Check sheet for the modelled part. Datum: model origin and axes. Units: mm. Face numbers are marked on the shaded views. A direction names the side the tool comes from. Give positions to 0.01 mm unless a question says otherwise; leave off trailing zeros. Order: outer loops, then holes, each group sorted by start corner. A loop starts at its lowest first (then second) coordinate and runs counter-clockwise, first axis right, second up.
Item 1: Release check for a two-part mould opening along X. For the marked faces 1 and 2 record: released by +X, released by -X, zero draft, split by the parting line, or undercut.
Item 2: Material ranges on line 1 along Y through (x, z) = (10, 1.7); line 2 along X through (y, z) = (-0.5, 1.25); line 3 along X through (y, z) = (2, 2.25), recorded low to high.
Item 3: Sectioned sample at C-C on y = 0. Count the separate pieces of the cut face and the enclosed holes in it, and give its area (3 significant figures).
Item 4: Gauge pin test, flat ends, axial feed: P1, Ø0.5, axis at x = 2.5, z = 1.5, coming from the +Y side; P2, Ø4, axis at x = 10, y = 0, coming from the +Z side; P3, Ø0.9, axis at x = 6.5, z = 2, coming from the -Y side. Record the tip position at first contact, or that the pin passes through.
Item 5: Sectioned sample at A-A on x = -1.5. Record the boundary of the cut face in (y, z).
Item 6: Sectioned sample at D-D on z = 6.25. Record the boundary of the cut face in (x, y).
Item 7: Sectioned sample at B-B on x = 10. Record the boundary of the cut face in (y, z).
Item 8: Access from +Z, -Z, +X, -X, +Y, -Y to the whole of each face (thin tool, end or side, straight path). Record for the marked faces 3 and 4.
from build123d import *

# Parameters (mm, degrees)
SKETCH_W        = 30
SKETCH_H        = 15
PAD_DEPTH       = 1
SKETCH001_W     = 27.8
SKETCH001_H     = 12.8
SKETCH001_W_2   = 25.8
SKETCH001_H_2   = 10.8
PAD001_DEPTH    = 1.8
SKETCH002_W     = 8
SKETCH002_H     = 1.1
PAD002_DEPTH    = 6
SKETCH003_W     = 5.2
SKETCH003_H     = 1
POCKET_DEPTH    = 28.901
SKETCH004_R     = 2.6
SKETCH004_R_2   = 1.6
PAD003_DEPTH    = 2.4
SKETCH005_W     = 10
SKETCH005_H     = 6
POCKET001_DEPTH = 5
CHAMFER_SIZE    = 0.5
CHAMFER001_SIZE = 0.5
CHAMFER002_SIZE = 0.5


with BuildPart() as part:
    # Sketch → Pad (new body)
    with BuildSketch(Plane.XY):
        Rectangle(SKETCH_W, SKETCH_H)
    extrude(amount=PAD_DEPTH)

    # Sketch001 → Pad001 (new body)
    with BuildSketch(Plane.XY.offset(1)):
        Rectangle(SKETCH001_W, SKETCH001_H)
        Rectangle(SKETCH001_W_2, SKETCH001_H_2, mode=Mode.SUBTRACT)
    extrude(amount=PAD001_DEPTH)

    # Sketch002 → Pad002 (new body)
    with BuildSketch(Plane.XY.offset(1)):
        with Locations((0, -6.95)):
            Rectangle(SKETCH002_W, SKETCH002_H)
    extrude(amount=PAD002_DEPTH)

    # Sketch003 → Pocket (cut, through all)
    with BuildSketch(Plane(origin=(-13.9, 0, 0), x_dir=(0, -1, 0), z_dir=(-1, 0, 0))):
        with Locations((0, 1.5)):
            Rectangle(SKETCH003_W, SKETCH003_H)
    extrude(amount=-POCKET_DEPTH, mode=Mode.SUBTRACT)

    # Sketch004 → Pad003 (new body)
    with BuildSketch(Plane.XY.offset(1)):
        with Locations((-10, 0)):
            Circle(SKETCH004_R)
        with Locations((-10, 0)):
            Circle(SKETCH004_R_2, mode=Mode.SUBTRACT)
        with Locations((10, 0)):
            Circle(SKETCH004_R)
        with Locations((10, 0)):
            Circle(SKETCH004_R_2, mode=Mode.SUBTRACT)
    extrude(amount=PAD003_DEPTH)

    # Sketch005 → Pocket001 (cut)
    with BuildSketch(Plane(origin=(0, 0, 0), x_dir=(1, 0, 0), z_dir=(0, 0, -1))):
        with Locations((0, -2)):
            Rectangle(SKETCH005_W, SKETCH005_H)
    extrude(amount=-POCKET001_DEPTH, mode=Mode.SUBTRACT)

    # Chamfer
    chamfer_edges = [part.edges().sort_by_distance(p)[0] for p in [
        (-11.6, 0, 3.4),
        (8.4, 0, 3.4),
    ]]
    chamfer(chamfer_edges, length=CHAMFER_SIZE)

    # Chamfer001
    chamfer001_edges = [part.edges().sort_by_distance(p)[0] for p in [
        (-13.9, 6.4, 1.9),
        (-13.9, 0, 2.8),
        (-13.9, -6.4, 1.9),
        (13.9, 6.4, 1.9),
        (13.9, 0, 2.8),
        (13.9, -6.4, 1.9),
    ]]
    chamfer(chamfer001_edges, length=CHAMFER001_SIZE)

    # Chamfer002
    chamfer002_edges = [part.edges().sort_by_distance(p)[0] for p in [
        (-5, 2, 0),
        (0, 5, 0),
        (5, 2, 0),
        (0, -1, 0),
    ]]
    chamfer(chamfer002_edges, length=CHAMFER002_SIZE)


solid = part.part
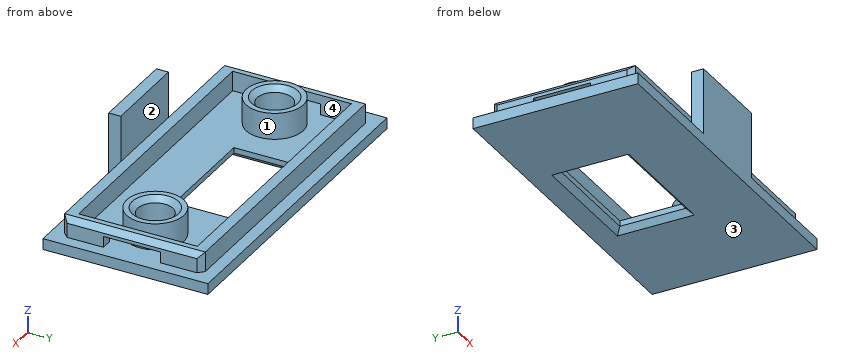
Report:
1. face 1: undercut
1. face 2: zero draft
2. line 1: y = -6.4 to -5.4, -2.6 to -1.6, 1.6 to 2.6, 5.4 to 6.4
2. line 2: x = -12.55 to -11.52, -8.48 to -7.45, 7.45 to 8.48, 11.52 to 12.55
2. line 3: x = -13.9 to -12.9, -11.66 to -8.34, 8.34 to 11.66, 12.9 to 13.9
3. separate pieces: 4
3. enclosed holes: 0
3. area: 30.2 mm2
4. P1: stops at y = 6.4
4. P2: stops at z = 3.3
4. P3: stops at y = -6.4
5. outline: (-7.5, 0) - (-1.5, 0) - (-1, 0.5) - (-1, 1) - (-5.4, 1) - (-5.4, 2.8) - (-6.4, 2.8) - (-6.4, 7) - (-7.5, 7) - close; (5, 0.5) - (5.5, 0) - (7.5, 0) - (7.5, 1) - (6.4, 1) - (6.4, 2.8) - (5.4, 2.8) - (5.4, 1) - (5, 1) - close
6. outline: (-4, -7.5) - (4, -7.5) - (4, -6.4) - (-4, -6.4) - close
7. outline: (-7.5, 0) - (7.5, 0) - (7.5, 1) - (6.4, 1) - (6.4, 2.8) - (5.4, 2.8) - (5.4, 1) - (2.6, 1) - (2.6, 3.4) - (2.1, 3.4) - (1.6, 2.9) - (1.6, 1) - (-1.6, 1) - (-1.6, 2.9) - (-2.1, 3.4) - (-2.6, 3.4) - (-2.6, 1) - (-5.4, 1) - (-5.4, 2.8) - (-6.4, 2.8) - (-6.4, 1) - (-7.5, 1) - close
8. face 3: -Z, +X, -X, +Y, -Y
8. face 4: +Z
